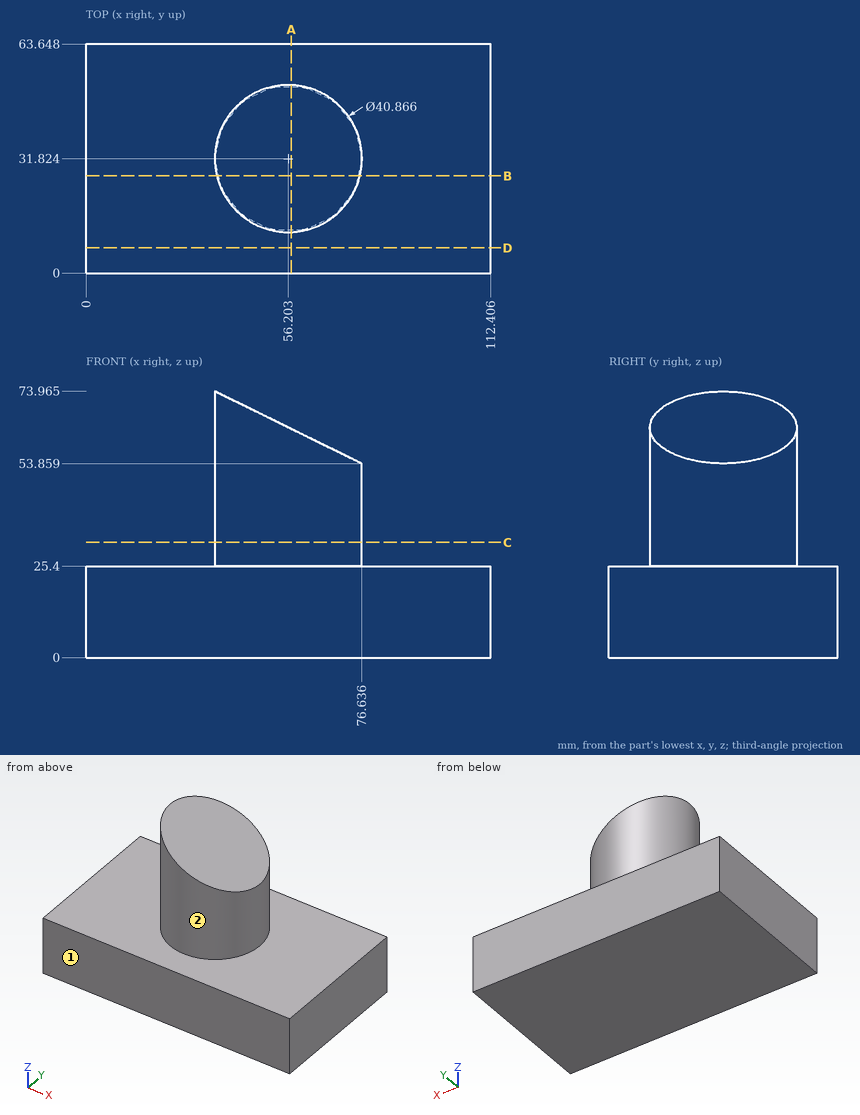
Can you work these out from the drawing? Everything is in mm from the part's minimum corner. A direction names the side the tool comes from. Round coordinates to 2 decimals unless told otherwise and drop trailing zeros. Order: outer loops, then holes, each group sorted by start corner. A loop starts at its lowest first (then second) coordinate and runs counter-clockwise, first axis right, second up. Notation, with made-up numbers: (25, 15.25) -> (30, 15.25) arc R13 cw to (30, 20.25) -> close; hole circle Ø1 at (43.25, 62). An arc over 180 degrees is marked (long way). Return JSON: item names as keys, results as strings. Group by question number.
1. If we section it at C-C, the plane z = 32: Write out the boundary of the cut face in (x, y), then the cut area to 3 significant figures.
2. Will these pins go through, and if not, where does the flat tip stop? pin 1 (6 mm diameter, centred on y = 25.5, z = 35.5, fed in from -X); pin 2 (8 mm diameter, centred on x = 83.5, z = 14.5, fed in from -Y); pin 3 (1 mm diameter, centred on x = 39, z = 57.5, fed in from -Y) (1 decimal); pin 4 (1.5 mm diameter, centred on x = 69.5, y = 40.5, fed in from +Z).
3. I need wall thicknesses on line 1 (Z direction, x = 98, y = 36); line 2 (X direction, y = 32.5, z = 27.5) (1 decimal); line 3 (Z direction, x = 53.5, y = 36.5). Which ranges of each line are inside material? Lowest first, please. Write a range as [from, to].
4. If we section it at D-D, the plane y = 7: Write out the boundary of the cut face in (x, z).
5. If we section it at B-B, the plane y = 27: Write out the boundary of the cut face in (x, z).
6. If we section it at A-A, the plane x = 57: Write out the boundary of the cut face in (y, z), then the cut area to 3 significant figures.
7. Which directions (+Z, -Z, +X, -X, +Y, -Y) give clear straight access to the entire face, cutting with the end or side of a thin tool? Please do the marked faces 1 and 2.
Output values:
{
 "1": {"outline": "circle Ø40.87 at (56.2, 31.82)", "area": "1,310 mm²"},
 "2": {"pin 1": "x = 36.04", "pin 2": "y = 0", "pin 3": "y = 20.1", "pin 4": "z = 57.74"},
 "3": {"line 1": "[0, 25.4]", "line 2": "[35.8, 76.6]", "line 3": "[0, 65.24]"},
 "4": {"outline": "(0, 0) -> (112.41, 0) -> (112.41, 25.4) -> (0, 25.4) -> close"},
 "5": {"outline": "(0, 0) -> (112.41, 0) -> (112.41, 25.4) -> (76.06, 25.4) -> (76.06, 54.14) -> (36.35, 73.68) -> (36.35, 25.4) -> (0, 25.4) -> close"},
 "6": {"outline": "(0, 0) -> (63.65, 0) -> (63.65, 25.4) -> (52.24, 25.4) -> (52.24, 63.52) -> (11.41, 63.52) -> (11.41, 25.4) -> (0, 25.4) -> close", "area": "3,170 mm²"},
 "7": {"face 1": "+Z, -Z, +X, -X, -Y", "face 2": "+Z"}
}
